```python
from build123d import *

# Parameters (mm, degrees)
ESQUISSE1_W        = 155
ESQUISSE1_H        = 90
ESQUISSE1_R        = 25
ESQUISSE1_R_2      = 2
ESQUISSE1_R_3      = 1.5
ESQUISSE1_R_4      = 2.9
BOSS_EXTRU_1_DEPTH = 3


with BuildPart() as part:
    # Esquisse1 → Boss.-Extru.1 (new body)
    with BuildSketch(Plane(origin=(0, 0, 0), x_dir=(1, 0, 0), z_dir=(0, 1, 0))):
        Rectangle(ESQUISSE1_W, ESQUISSE1_H)
        with Locations(Location((-37.5, 0, 0), (0, 0, 270))):
            Circle(ESQUISSE1_R, mode=Mode.SUBTRACT)
        with Locations(Location((-64.5, 27, 0), (0, 0, 270))):
            Circle(ESQUISSE1_R_2, mode=Mode.SUBTRACT)
        with Locations(Location((-10.5, 27, 0), (0, 0, 90))):
            Circle(ESQUISSE1_R_2, mode=Mode.SUBTRACT)
        with Locations(Location((-10.5, -27, 0), (0, 0, 270))):
            Circle(ESQUISSE1_R_2, mode=Mode.SUBTRACT)
        with Locations(Location((-64.5, -27, 0), (0, 0, 90))):
            Circle(ESQUISSE1_R_2, mode=Mode.SUBTRACT)
        with Locations(Location((10.5, -27, 0), (0, 0, 90))):
            Circle(ESQUISSE1_R_2, mode=Mode.SUBTRACT)
        with Locations(Location((64.5, -27, 0), (0, 0, 270))):
            Circle(ESQUISSE1_R_2, mode=Mode.SUBTRACT)
        with Locations(Location((64.5, 27, 0), (0, 0, 90))):
            Circle(ESQUISSE1_R_2, mode=Mode.SUBTRACT)
        with Locations(Location((10.5, 27, 0), (0, 0, 270))):
            Circle(ESQUISSE1_R_2, mode=Mode.SUBTRACT)
        with Locations(Location((37.5, 0, 0), (0, 0, 90))):
            Circle(ESQUISSE1_R, mode=Mode.SUBTRACT)
        with Locations(Location((-73, 40.5, 0), (0, 0, 270))):
            Circle(ESQUISSE1_R_3, mode=Mode.SUBTRACT)
        with Locations(Location((73, 40.5, 0), (0, 0, 90))):
            Circle(ESQUISSE1_R_3, mode=Mode.SUBTRACT)
        with Locations(Location((73, -40.5, 0), (0, 0, 270))):
            Circle(ESQUISSE1_R_3, mode=Mode.SUBTRACT)
        with Locations(Location((-73, -40.5, 0), (0, 0, 90))):
            Circle(ESQUISSE1_R_3, mode=Mode.SUBTRACT)
        with Locations(Location((-7, 39, 0), (0, 0, 270))):
            Circle(ESQUISSE1_R_4, mode=Mode.SUBTRACT)
        with Locations(Location((7, 39, 0), (0, 0, 90))):
            Circle(ESQUISSE1_R_4, mode=Mode.SUBTRACT)
    extrude(amount=BOSS_EXTRU_1_DEPTH)


solid = part.part
```
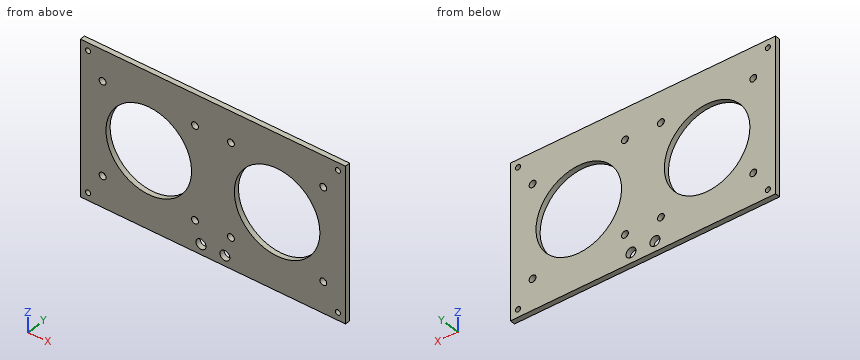
The listing builds one solid part. Answer for the finished solid, in the listing's coordinates (mm). Round coordinates to 2 decimals unless told otherwise and drop trailing zeros. Loops run counter-clockwise (first coordinate to the right, second up) from the corner with the lowest first, then second, coordinate; pieces in that order, holes last.
Q1. Given pin 1 Ø2.5 at (x, z) = (-73, -40.5) entering from +Y, flat-ended and moving along its own axis, determine where the tip first touches the part or whether it passes through.
Q2. Find the intervals of material crossed by line 1 (X direction, y = 1.3, z = 0); line 2 (Z direction, x = -73, y = 1.25); line 3 (X direction, y = 1.8, z = 27), in increasing order.
Q3. Section A-A, the plane z = 27 is taken. Determine the outline of the cut face in (x, y).
Q4. Section D-D, the plane z = -1 is taken. Determine the outline of the cut face in (x, y).
Q5. Section C-C, the plane y = 2.55 is taken. Count the separate pieces of the cut face and the enclosed holes in it, then the cut area to 3 significant figures.
Q6. Section B-B, the plane x = -73 is taken. Determine the outline of the cut face in (y, z).
Completed:
1. pin 1: passes through
2. line 1: x = -77.5 to -62.5, -12.5 to 12.5, 62.5 to 77.5
2. line 2: z = -45 to -42, -39 to 39, 42 to 45
2. line 3: x = -77.5 to -66.5, -62.5 to -12.5, -8.5 to 8.5, 12.5 to 62.5, 66.5 to 77.5
3. outline: (-77.5, 0) - (-66.5, 0) - (-66.5, 3) - (-77.5, 3) - close; (-62.5, 0) - (-12.5, 0) - (-12.5, 3) - (-62.5, 3) - close; (-8.5, 0) - (8.5, 0) - (8.5, 3) - (-8.5, 3) - close; (12.5, 0) - (62.5, 0) - (62.5, 3) - (12.5, 3) - close; (66.5, 0) - (77.5, 0) - (77.5, 3) - (66.5, 3) - close
4. outline: (-77.5, 0) - (-62.48, 0) - (-62.48, 3) - (-77.5, 3) - close; (-12.52, 0) - (12.52, 0) - (12.52, 3) - (-12.52, 3) - close; (62.48, 0) - (77.5, 0) - (77.5, 3) - (62.48, 3) - close
5. separate pieces: 1
5. enclosed holes: 16
5. area: 9,840 mm2
6. outline: (0, -45) - (3, -45) - (3, -42) - (0, -42) - close; (0, -39) - (3, -39) - (3, 39) - (0, 39) - close; (0, 42) - (3, 42) - (3, 45) - (0, 45) - close
